Design review of the part built by this model. Coordinates are the model's own, in mm. Coordinates: 2 decimals unless noted, no trailing zeros. Write each loop counter-clockwise with the first axis right and the second up, starting at its lowest first coordinate (ties: lowest second). Pieces come first, ordered by that corner, then holes. Notation, with made-up numbers: (23, 43) - (70, 43) arc R31 ccw to (70, 77) - close; hole circle Ø10 at (25.5, 51.5). An arc over 180 degrees is marked (long way). Use a Markdown table: item, result.
from build123d import *

# Parameters (mm, degrees)
F1_DEPTH = 6
F2_D     = 11


with BuildPart() as f1:
    # F0 (on Front) → F1 (new body)
    with BuildSketch(Plane.XZ):
        with BuildLine():
            Line((266.2244143939, 186.4123418141), (307.1820166084, 215.0911636316))
            ThreePointArc((307.1820166084, 215.0911636316), (0, 375), (-307.1820166084, 215.0911636316))
            Line((-307.1820166084, 215.0911636316), (-266.2244143939, 186.4123418141))
            ThreePointArc((-266.2244143939, 186.4123418141), (0, 325), (266.2244143939, 186.4123418141))
        make_face()
    extrude(amount=F1_DEPTH)

    # F2 (through all)
    with Locations(Plane(origin=(0, 0, 0), x_dir=(1, 0, 0), z_dir=(0, 1, 0))):
        with Locations((-224.9756633903, -268.1155550916), (-119.707050164, -328.8924172751), (119.707050164, -328.8924172751), (224.9756633903, -268.1155550916)):
            Hole(F2_D / 2)


solid = f1.part
(1) For pin 1 (9 mm diameter, centred on x = -119.71, z = 328.89, fed in from -Y); pin 2 (14.5 mm diameter, centred on x = 224.98, z = 268.12, fed in from +Y); pin 3 (3 mm diameter, centred on y = -2, z = 237, fed in from -X); pin 4 (2 mm diameter, centred on x = -161.5, y = -4.5, fed in from +Z), all flat-tipped, find the tip position at first contact; note any pin that passes through.
Determined:
| item | result |
|---|---|
| pin 1 | through |
| pin 2 | y = 0 |
| pin 3 | x = -291.83 |
| pin 4 | z = 338.92 |
(2) Take a section at A-A on z = 294. Write out the cut boundary in (x, y), and give its area (3 significant figures).
Determined:
| item | result |
|---|---|
| outline | (-232.79, -6) - (-138.52, -6) - (-138.52, 0) - (-232.79, 0) - close; (138.52, -6) - (232.79, -6) - (232.79, 0) - (138.52, 0) - close |
| area | 1,130 mm2 |
(3) Take a section at D-D on z = 199. Write out the cut boundary in (x, y), and give its area (3 significant figures).
Determined:
| item | result |
|---|---|
| outline | (-284.2, -6) - (-256.95, -6) - (-256.95, 0) - (-284.2, 0) - close; (256.95, -6) - (284.2, -6) - (284.2, 0) - (256.95, 0) - close |
| area | 327 mm2 |
(4) Take a section at C-C on z = 360. Write out the cut boundary in (x, y).
Determined:
| item | result |
|---|---|
| outline | (-105, -6) - (105, -6) - (105, 0) - (-105, 0) - close |
(5) Draft analysis for pull direction X (two halves, no side actions). For faces 1 (the flat face through (-286.99, -2.958, 200.953)), 2 (the cylindrical face through (-219.48, -3.04, 267.87)), 3 (the cylindrical face through (-118.99, -3.04, 323.44)), 4 (the cylindrical face through (5.039, -2.958, 374.966)), state which applies: +X half, -X half, draft (parallel to the pull), parting line (faces both ways), or undercut.
Determined:
| item | result |
|---|---|
| face 1 | -X half |
| face 2 | undercut |
| face 3 | undercut |
| face 4 | parting line |
(6) Take a section at B-B on y = -1.9. Write out the cut boundary in (x, z).
Determined:
| item | result |
|---|---|
| outline | (-307.18, 215.09) - (-266.22, 186.41) arc R325 cw to (266.22, 186.41) - (307.18, 215.09) arc R375 ccw to start; hole circle Ø11 at (-224.98, 268.12); hole circle Ø11 at (-119.71, 328.89); hole circle Ø11 at (119.71, 328.89); hole circle Ø11 at (224.98, 268.12) |
(7) For L1, parallel to X at y = -3.25, z = 204.5; L2, parallel to X at y = -2.9, z = 243; L3, parallel to Z at x = 221.5, y = -3.45, list the stretches that pass through material, from the lowest coordinate up. Write a range as from..to.
Determined:
| item | result |
|---|---|
| L1 | -292.06..-252.6, 252.6..292.06 |
| L2 | -285.62..-215.81, 215.81..285.62 |
| L3 | 237.83..263.85, 272.38..302.59 |
